Can you work these out from the model? Positions are in its coordinate system, mm. Face numbers are marked on the shaded views. A direction names the side the tool comes from. Give positions to 0.01 mm unless a question says otherwise; leave off trailing zeros. Order: outer loops, then holes, each group sorted by start corner. A loop starts at its lowest first (then second) coordinate and runs counter-clockwise, first axis right, second up. Notation, with made-up numbers: (-4, 72.5) -> (0, 72.5) arc R28 cw to (0, 99.5) -> close; hole circle Ø1 at (81, -6.75). An arc over 180 degrees is marked (long way). Answer as CSV lines item,"result".
```python
from build123d import *

# Parameters (mm, degrees)
F0_R     = 11
F0_R_2   = 10
F1_DEPTH = 17
F2_R     = 15
F3_DEPTH = 9.75
F4_R     = 7
F6_R     = 11.25
F6_R_2   = 11
F7_DEPTH = 13
F8_R     = 4.2
F9_DEPTH = 25.4


with BuildPart() as f1:
    # F0 (on Top) → F1 (new body)
    with BuildSketch(Plane.XY):
        Circle(F0_R)
        Circle(F0_R_2, mode=Mode.SUBTRACT)
    extrude(amount=F1_DEPTH)

    # F2 (on face) → F3 (join)
    with BuildSketch(Plane.XY.offset(17)):
        Circle(F2_R)
    extrude(amount=F3_DEPTH)

    # F4
    f4_edges = [f1.edges().sort_by_distance(p)[0] for p in [
        (-15, 0, 26.75),
    ]]
    fillet(f4_edges, radius=F4_R)

    # F6 (on offset) → F7 (join, through all)
    with BuildSketch(Plane(origin=(0, 0, 4), x_dir=(1, 0, 0), z_dir=(0, 0, -1))):
        Circle(F6_R)
        Circle(F6_R_2, mode=Mode.SUBTRACT)
    extrude(amount=-F7_DEPTH)

    # F8 (on face) → F9 (cut)
    with BuildSketch(Plane.XY.offset(26.75)):
        Circle(F8_R)
    extrude(amount=-F9_DEPTH, mode=Mode.SUBTRACT)


solid = f1.part
```
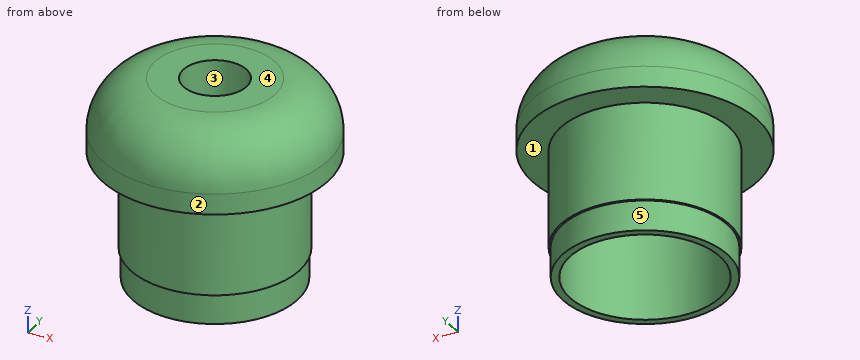
Item 1: We'd pull the mould along Y, two halves only. Please class the marked faces 3, 4 and 5: released by +Y, released by -Y, zero draft, split by the parting line, or undercut.
Numbers:
face 3,"undercut"
face 4,"zero draft"
face 5,"split by the parting line"
Item 2: Imagine slicing it at C-C, the plane z = 3.5. Please give me the cut outline in (x, y), then the cut area to 3 significant figures.
Numbers:
outline,"circle Ø22 at (0, 0); hole circle Ø20 at (0, 0)"
area,"66.0 mm²"
Item 3: Imagine slicing it at D-D, the plane z = 14.75. Please give me the cut outline in (x, y).
Numbers:
outline,"circle Ø22.5 at (0, 0); hole circle Ø20 at (0, 0)"
Item 4: For pin 1 (3 mm diameter, centred on x = -4.5, y = -3.5, fed in from -Z); pin 2 (6.5 mm diameter, centred on x = 0, y = 0, fed in from -Z); pin 3 (5 mm diameter, centred on x = 7, z = 24, fed in from +Y); pin 4 (4 mm diameter, centred on y = -3.5, z = 12.5, fed in from -X), each with a flat end and sliding along its axis, tell me the tip position at first contact or that it passes through.
Numbers:
pin 1,"stops at z = 17"
pin 2,"passes through"
pin 3,"stops at y = 13.57"
pin 4,"stops at x = -11.15"
Item 5: Imagine slicing it at A-A, the plane y = 0. Please give me the cut outline in (x, z).
Numbers:
outline,"(-15, 17) -> (-11.25, 17) -> (-11.25, 4) -> (-11, 4) -> (-11, 0) -> (-10, 0) -> (-10, 17) -> (-4.2, 17) -> (-4.2, 26.75) -> (-8, 26.75) arc R7 ccw to (-15, 19.75) -> close; (4.2, 17) -> (10, 17) -> (10, 0) -> (11, 0) -> (11, 4) -> (11.25, 4) -> (11.25, 17) -> (15, 17) -> (15, 19.75) arc R7 ccw to (8, 26.75) -> (4.2, 26.75) -> close"
Item 6: For the marked faces 1 and 2, which set-ups out of +Z, -Z, +X, -X, +Y, -Y let a thin tool reach every point of the face, with its end or its side?
Numbers:
face 1,"-Z"
face 2,"+Z, -Z"
Item 7: Please list where these lines run through material, in increasing order: line 1 along Y through (x, z) = (0, 20); line 2 along Y through (x, z) = (0, 6.5); line 3 along Z through (x, y) = (-4.75, -2.5).
Numbers:
line 1,"y = -15 to -4.2, 4.2 to 15"
line 2,"y = -11.25 to -10, 10 to 11.25"
line 3,"z = 17 to 26.75"
